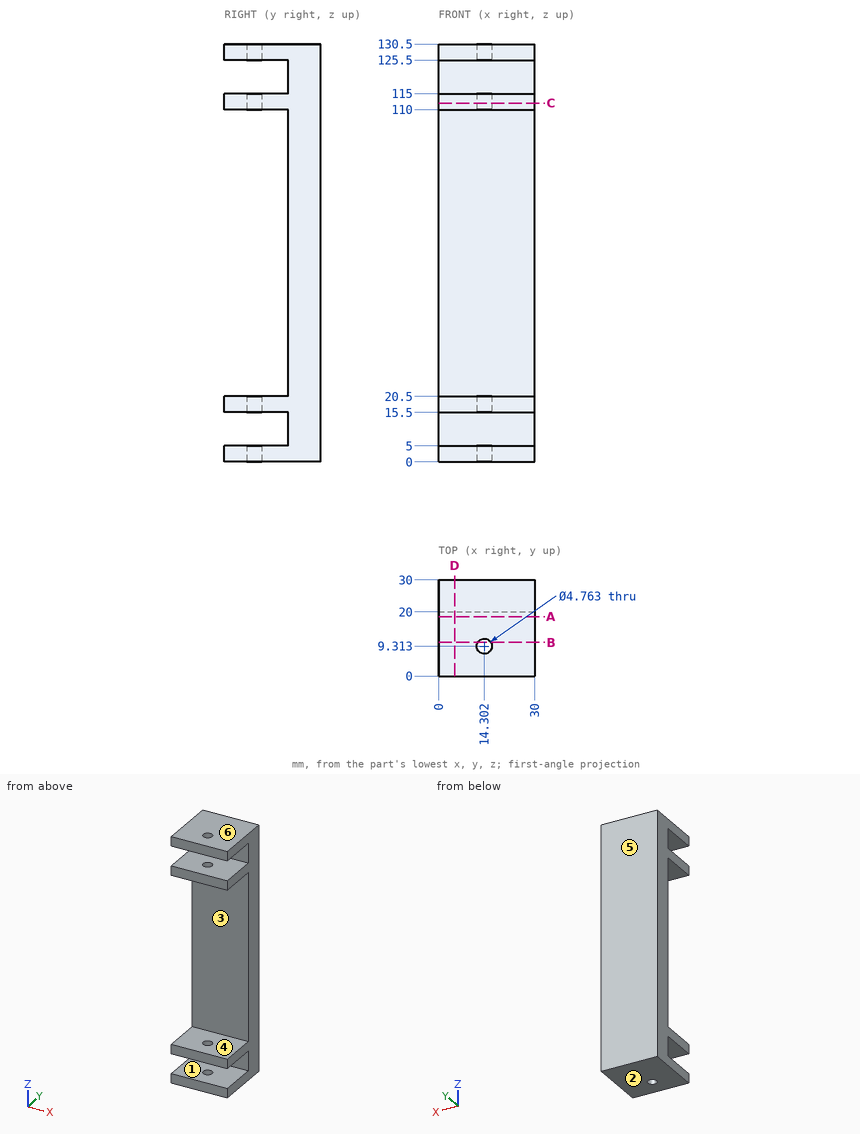
Job drawing, mm, ordinate dimensions from the low corner. One solid piece. A direction names the side the tool comes from. Coordinates: 2 decimals unless noted, no trailing zeros. Order: outer loops, then holes, each group sorted by start corner. A loop starts at its lowest first (then second) coordinate and runs counter-clockwise, first axis right, second up. Notation, with made-up numbers: (-26, 80) - (17, 80) arc R12 cw to (17, 84) - close; hole circle Ø1 at (0.25, 70.25). An arc over 180 degrees is marked (long way). Return JSON: item names as keys, results as strings. Group by question number.
1) Saw through at A-A, the plane y = 18.5. Write the cut outline in (x, z).
2) Mould opens along Z. For the marked faces 3, 4, 5 and 6 say: released by +Z, released by -Z, zero draft, split by the parting line, or undercut.
3) Tool access for the marked faces 1 and 2: list every direction of +Z, -Z, +X, -X, +Y, -Y with a clear straight run to the whole face (end or side of a thin tool).
4) Probe line 1 (Z direction, x = 11.5, y = 10.5); line 2 (Y direction, x = 14, z = 101). List the from-to ranges inside material, lowest first. Write a range as from..to.
5) Saw through at B-B, the plane y = 10.5. Count the separate pieces of the cut face and the enclosed holes in it.
6) Saw through at D-D, the plane x = 5. Write the cut outline in (y, z), plus the area to 4 significant figures.
7) Saw through at C-C, the plane z = 112. Write the cut outline in (x, y).
8) Flat gauge pins, fed straight in: P1, Ø6, axis at x = 14.5, y = 8.5, coming from the -Z side; P2, Ø3, axis at x = 19, z = 120.5, coming from the -Y side. Where does each tip first touch, or does it go through?
Values found:
{
 "1": {"outline": "(0, 0) - (30, 0) - (30, 5) - (0, 5) - close; (0, 15.5) - (30, 15.5) - (30, 20.5) - (0, 20.5) - close; (0, 110) - (30, 110) - (30, 115) - (0, 115) - close; (0, 125.5) - (30, 125.5) - (30, 130.5) - (0, 130.5) - close"},
 "2": {"face 3": "undercut", "face 4": "undercut", "face 5": "zero draft", "face 6": "released by +Z"},
 "3": {"face 1": "+X, -X, -Y", "face 2": "-Z, +X, -X, +Y, -Y"},
 "4": {"line 1": "z = 0..5, 15.5..20.5, 110..115, 125.5..130.5", "line 2": "y = 20..30"},
 "5": {"separate pieces": "8", "enclosed holes": "0"},
 "6": {"outline": "(0, 0) - (30, 0) - (30, 130.5) - (0, 130.5) - (0, 125.5) - (20, 125.5) - (20, 115) - (0, 115) - (0, 110) - (20, 110) - (20, 20.5) - (0, 20.5) - (0, 15.5) - (20, 15.5) - (20, 5) - (0, 5) - close", "area": "1,705 mm²"},
 "7": {"outline": "(0, 0) - (30, 0) - (30, 30) - (0, 30) - close; hole circle Ø4.76 at (14.3, 9.31)"},
 "8": {"P1": "stops at z = 0", "P2": "stops at y = 20"}
}
